Source: CAD feature listing. Evaluate the final solid. Frame: model axes, mm. A direction names the side the tool comes from. Give positions to 0.01 mm unless a question says otherwise; leave off trailing zeros. Loops run counter-clockwise (first coordinate to the right, second up) from the corner with the lowest first, then second, coordinate; pieces in that order, holes last. Notation, with made-up numbers: M 72.5,31.25 L 95.5,31.25 A21 cw 95.5,67.25 Z; hole C 13,-16 d3. An arc over 180 degrees is marked long. Answer in a Markdown table with one row per item.
```python
from build123d import *

# Parameters (mm, degrees)
SKETCH_5_W                = 42.3
SKETCH_5_H                = 50.3
SKETCH_5_R                = 11.15
SKETCH_5_R_2              = 2.15
EXTRUDE_2_DEPTH           = 4
EXTRUDE_3_DEPTH           = 4
SKETCH_7_R                = 1.7
CUT_EXTRUDE_3_DEPTH       = 4
CHAMFER_1_SIZE            = 4
EXTRUDE_4_DEPTH           = 2
EXTRUDE_5_REACH           = 79.8
EXTRUDE_6_REACH           = 80.956
SKETCH_12_W               = 46.3
SKETCH_12_H               = 3
EXTRUDE_7_DEPTH           = 53
EXTRUDE_9_DEPTH           = 4
CUT_EXTRUDE_4_DEPTH       = 5
SKETCH_17_R               = 5.175
EXTRUDE_10_DEPTH          = 15
SKETCH_18_R               = 1.6
CUT_EXTRUDE_6_DEPTH       = 15
F_2_0MM_1_D               = 3.1
F_2_0MM_1_DEPTH           = 4.45
F_2_0MM_1_TIP             = 1.55
F_2_0MM_1_ON_FACE_2_D     = 3.1
F_2_0MM_1_ON_FACE_2_DEPTH = 4.45
F_2_0MM_1_ON_FACE_2_TIP   = 1.55
F_2_0MM_1_ON_FACE_3_D     = 3.1
F_2_0MM_1_ON_FACE_3_DEPTH = 4.45
F_2_0MM_1_ON_FACE_3_TIP   = 1.55
SKETCH_21_W               = 46.3
SKETCH_21_H               = 53
CUT_EXTRUDE_7_DEPTH       = 1.5
CUT_EXTRUDE_START         = -0.5
CUT_EXTRUDE_8_DEPTH       = 0.5
EXTRUDE_START             = 2.5
EXTRUDE_11_DEPTH          = 2.5


with BuildPart() as part:
    # Sketch 5 → Extrude 2 (new body)
    with BuildSketch(Plane.XY):
        with Locations((0, 25.15)):
            Rectangle(SKETCH_5_W, SKETCH_5_H)
        with Locations((0, 29.15)):
            Circle(SKETCH_5_R, mode=Mode.SUBTRACT)
        with Locations((15.5, 44.65)):
            Circle(SKETCH_5_R_2, mode=Mode.SUBTRACT)
        with Locations(Location((15.5, 13.65, 0), (0, 0, 180))):
            Circle(SKETCH_5_R_2, mode=Mode.SUBTRACT)
        with Locations((-15.5, 13.65)):
            Circle(SKETCH_5_R_2, mode=Mode.SUBTRACT)
        with Locations(Location((-15.5, 44.65, 0), (0, 0, 180))):
            Circle(SKETCH_5_R_2, mode=Mode.SUBTRACT)
    extrude(amount=-EXTRUDE_2_DEPTH)

    # Sketch 6 → Extrude 3 (add)
    with BuildSketch(Plane.XZ):
        with BuildLine():
            Line((-21.15, 0), (-19.967256346, 20.643972909))
            ThreePointArc((-19.967256346, 20.643972909), (0, 39.5), (19.967256346, 20.643972909))
            Line((19.967256346, 20.643972909), (21.15, 0))
            Line((21.15, 0), (-21.15, 0))
        make_face()
    extrude(amount=-EXTRUDE_3_DEPTH)

    # Sketch 7 → Cut-Extrude 3 (cut)
    with BuildSketch(Plane(origin=(0, 4, 0), x_dir=(1, 0, 0), z_dir=(0, 1, 0))):
        with Locations(Location((0, -5.5, 0), (0, 0, 270))):
            Circle(SKETCH_7_R)
        with Locations(Location((12.124355653, -12.5, 0), (0, 0, 270))):
            Circle(SKETCH_7_R)
        with Locations(Location((12.124355653, -26.5, 0), (0, 0, 270))):
            Circle(SKETCH_7_R)
        with Locations(Location((0, -33.5, 0), (0, 0, 270))):
            Circle(SKETCH_7_R)
        with Locations(Location((-12.124355653, -26.5, 0), (0, 0, 270))):
            Circle(SKETCH_7_R)
        with Locations(Location((-12.124355653, -12.5, 0), (0, 0, 270))):
            Circle(SKETCH_7_R)
    extrude(amount=-CUT_EXTRUDE_3_DEPTH, mode=Mode.SUBTRACT)

    # Chamfer 1
    chamfer_1_edges = [part.edges().sort_by_distance(p)[0] for p in [
        (-21.15, 50.3, -2),
        (21.15, 50.3, -2),
    ]]
    chamfer(chamfer_1_edges, length=CHAMFER_1_SIZE)

    # Sketch 9 → Extrude 4 (add)
    with BuildSketch(Plane.ZY.offset(21.15)):
        Polygon((-4, 0), (8, 0), (2, 15.3), (-4, 15.3), align=None)
    extrude_4 = extrude(amount=EXTRUDE_4_DEPTH)

    # Extrude 5: up to this face of the body (flat: up to its plane)
    extrude_5_end = Plane(part.part.faces().sort_by_distance((-20.558628173, 2, 10.321986454))[0])
    # Sketch 10 → Extrude 5 (add, up to the picked face)
    with BuildSketch(Plane.ZY.offset(23.15), mode=Mode.PRIVATE) as extrude_5_sk1:
        Polygon((-4, 0), (8, 0), (6.431372549, 4), (-4, 4), align=None)
    extrude_5_tool1 = split(extrude(extrude_5_sk1.sketch, amount=-EXTRUDE_5_REACH, mode=Mode.PRIVATE), bisect_by=extrude_5_end, keep=Keep.BOTH, mode=Mode.PRIVATE)
    add(extrude_5_tool1.solids().sort_by(Axis((-23.15, 1.95338, 1.616984), (1, 0, 0)))[0])

    # Mirror 2: Extrude 4 across plane
    add(extrude_4.mirror(Plane(origin=(0, 0, 0), x_dir=(0, 0, 1), z_dir=(1, 0, 0))))

    # Extrude 6: up to this face of the body (flat: up to its plane)
    extrude_6_end = Plane(part.part.faces().sort_by_distance((20.558628173, 2, 10.321986454))[0])
    # Sketch 11 → Extrude 6 (add, up to the picked face)
    with BuildSketch(Plane(origin=(23.15, 0, 0), x_dir=(0, 0, -1), z_dir=(1, 0, 0)), mode=Mode.PRIVATE) as extrude_6_sk1:
        Polygon((-6.431372549, 4), (4, 4), (4, 0), (-8, 0), align=None)
    extrude_6_tool1 = split(extrude(extrude_6_sk1.sketch, amount=-EXTRUDE_6_REACH, mode=Mode.PRIVATE), bisect_by=extrude_6_end, keep=Keep.BOTH, mode=Mode.PRIVATE)
    add(extrude_6_tool1.solids().sort_by(Axis((23.15, 1.95338, 1.616984), (-1, 0, 0)))[0])

    # Sketch 12 → Extrude 7 (add)
    with BuildSketch(Plane(origin=(0, 0, -4), x_dir=(-1, 0, 0), z_dir=(0, 0, -1))):
        with Locations((0, 6.5)):
            Rectangle(SKETCH_12_W, SKETCH_12_H)
    extrude(amount=EXTRUDE_7_DEPTH)

    # Sketch 14 → Extrude 9 (add)
    with BuildSketch(Plane(origin=(0, 4, 0), x_dir=(1, 0, 0), z_dir=(0, 1, 0))):
        with BuildLine():
            Line((21.15, 0), (-21.15, 0))
            Line((-21.15, 0), (-21.15, -6.431372549))
            Line((-21.15, -6.431372549), (-20.781530951, -6.431372549))
            Line((-20.781530951, -6.431372549), (-19.967256346, -20.643972909))
            ThreePointArc((-19.967256346, -20.643972909), (0, -39.5), (19.967256346, -20.643972909))
            Line((19.967256346, -20.643972909), (20.781530951, -6.431372549))
            Line((20.781530951, -6.431372549), (21.15, -6.431372549))
            Line((21.15, -6.431372549), (21.15, 0))
        make_face()
    extrude(amount=EXTRUDE_9_DEPTH)

    # Sketch 15 → Cut-Extrude 4 (cut)
    with BuildSketch(Plane.XZ):
        with BuildLine():
            Line((-23.15, -4), (23.15, -4))
            Line((23.15, -4), (23.15, 8))
            Line((23.15, 8), (20.691660451, 8))
            Line((20.691660451, 8), (19.967256346, 20.643972909))
            ThreePointArc((19.967256346, 20.643972909), (0, 39.5), (-19.967256346, 20.643972909))
            Line((-19.967256346, 20.643972909), (-20.691660451, 8))
            Line((-20.691660451, 8), (-23.15, 8))
            Line((-23.15, 8), (-23.15, -4))
        make_face()
    extrude(amount=-CUT_EXTRUDE_4_DEPTH, mode=Mode.SUBTRACT)

    # Sketch 17 → Extrude 10 (add)
    with BuildSketch(Plane(origin=(0, 8, 0), x_dir=(1, 0, 0), z_dir=(0, 1, 0))):
        with Locations(Location((0, 16.5, 0), (0, 0, 270))):
            Circle(SKETCH_17_R)
    extrude(amount=-EXTRUDE_10_DEPTH)

    # Sketch 18 → Cut-Extrude 6 (cut)
    with BuildSketch(Plane.XZ.offset(7)):
        with Locations(Location((0, -16.5, 0), (0, 0, 270))):
            Circle(SKETCH_18_R)
    extrude(amount=-CUT_EXTRUDE_6_DEPTH, mode=Mode.SUBTRACT)

    # 2.0mm _1
    with Locations(Plane(origin=(-2.383959963, -1.470142013, -11.906813753), x_dir=(0.887572221549, 0, 0.46066859187), z_dir=(-0.46066859187, 0, 0.887572221549))):
        with Locations((0, 0)):
            Hole(F_2_0MM_1_D / 2, depth=F_2_0MM_1_DEPTH)
            with Locations((0, 0, -(F_2_0MM_1_DEPTH + F_2_0MM_1_TIP / 2))):  # 90° drill point
                Cone(0, F_2_0MM_1_D / 2, F_2_0MM_1_TIP, mode=Mode.SUBTRACT)

    # 2.0mm _1 on face 2
    with Locations(Plane(origin=(-4.001379199, -1.359919587, -19.781705274), x_dir=(0.634146160856, 0, -0.773213196131), z_dir=(-0.773213196131, 0, -0.634146160856))):
        with Locations((-1e-09, 0)):
            Hole(F_2_0MM_1_ON_FACE_2_D / 2, depth=F_2_0MM_1_ON_FACE_2_DEPTH)
            with Locations((0, 0, -(F_2_0MM_1_ON_FACE_2_DEPTH + F_2_0MM_1_ON_FACE_2_TIP / 2))):  # 90° drill point
                Cone(0, F_2_0MM_1_ON_FACE_2_D / 2, F_2_0MM_1_ON_FACE_2_TIP, mode=Mode.SUBTRACT)

    # 2.0mm _1 on face 3
    with Locations(Plane(origin=(4.74207792, -1.268589172, -18.572033301), x_dir=(0.40039282367, 0, 0.916343596449), z_dir=(0.916343596449, 0, -0.40039282367))):
        with Locations((0, 0)):
            Hole(F_2_0MM_1_ON_FACE_3_D / 2, depth=F_2_0MM_1_ON_FACE_3_DEPTH)
            with Locations((0, 0, -(F_2_0MM_1_ON_FACE_3_DEPTH + F_2_0MM_1_ON_FACE_3_TIP / 2))):  # 90° drill point
                Cone(0, F_2_0MM_1_ON_FACE_3_D / 2, F_2_0MM_1_ON_FACE_3_TIP, mode=Mode.SUBTRACT)

    # Sketch 21 → Cut-Extrude 7 (cut)
    with BuildSketch(Plane(origin=(0, 8, 0), x_dir=(1, 0, 0), z_dir=(0, 1, 0))):
        with Locations((0, 30.5)):
            Rectangle(SKETCH_21_W, SKETCH_21_H)
    extrude(amount=-CUT_EXTRUDE_7_DEPTH, mode=Mode.SUBTRACT)

    # Sketch 22 → Cut-Extrude 8 (cut)
    with BuildSketch(Plane(origin=(0, 8, 0), x_dir=(1, 0, 0), z_dir=(0, 1, 0)).offset(CUT_EXTRUDE_START)):
        with BuildLine():
            Line((21.15, -6.431372549), (21.15, -4.862745098))
            Line((21.15, -4.862745098), (21.15, 0))
            Line((21.15, 0), (-21.15, 0))
            Line((-21.15, 0), (-21.15, -4.862745098))
            Line((-21.15, -4.862745098), (-21.15, -6.431372549))
            Line((-21.15, -6.431372549), (-20.781530951, -6.431372549))
            Line((-20.781530951, -6.431372549), (-19.967256346, -20.643972909))
            ThreePointArc((-19.967256346, -20.643972909), (0, -39.5), (19.967256346, -20.643972909))
            Line((19.967256346, -20.643972909), (20.781530951, -6.431372549))
            Line((20.781530951, -6.431372549), (21.15, -6.431372549))
        make_face()
    extrude(amount=CUT_EXTRUDE_8_DEPTH, mode=Mode.SUBTRACT)

    # Sketch 23 → Extrude 11 (add)
    with BuildSketch(Plane.XZ.offset(-5).offset(EXTRUDE_START)):
        with BuildLine():
            Line((23.15, -57), (23.15, 6.039215686))
            Line((23.15, 6.039215686), (21.15, 6.039215686))
            Line((21.15, 6.039215686), (21.15, 6.431372549))
            Line((21.15, 6.431372549), (20.781530951, 6.431372549))
            Line((20.781530951, 6.431372549), (19.967256346, 20.643972909))
            ThreePointArc((19.967256346, 20.643972909), (0, 39.5), (-19.967256346, 20.643972909))
            Line((-19.967256346, 20.643972909), (-20.781530951, 6.431372549))
            Line((-20.781530951, 6.431372549), (-21.15, 6.431372549))
            Line((-21.15, 6.431372549), (-21.15, 6.039215686))
            Line((-21.15, 6.039215686), (-23.15, 6.039215686))
            Line((-23.15, 6.039215686), (-23.15, -57))
            Line((-23.15, -57), (23.15, -57))
        make_face()
    extrude(amount=-EXTRUDE_11_DEPTH)


solid = part.part
```
1) Pin query (flat end, axial travel): pin 1 Ø23 at (x, z) = (2, -42.5) entering from +Y; pin 2 Ø2 at (x, y) = (-22, 4) entering from +Z; pin 3 Ø2.5 at (x, z) = (0, -16.5) entering from +Y; pin 4 Ø3.5 at (x, y) = (15.5, 13.65) entering from -Z. Return the tip coordinate at first contact, or that it passes through.
Reply:
| item | result |
|---|---|
| pin 1 | stops at y = 6.5 |
| pin 2 | stops at z = 6.43 |
| pin 3 | stops at y = 5 |
| pin 4 | passes through |
2) Section D-D, the plane y = 44.65. Return loops of the section in (x, z).
Reply:
| item | result |
|---|---|
| outline | M -21.15,-4 L -17.65,-4 L -17.65,0 L -21.15,0 Z; M -13.35,-4 L 13.35,-4 L 13.35,0 L -13.35,0 Z; M 17.65,-4 L 21.15,-4 L 21.15,0 L 17.65,0 Z |
3) Pull-direction query (Y, two-part tool) for faces 6 (the flat face through (22, 4, 6.039)), 7 (the flat face through (0, 50.3, -2)), 8 (the cylindrical face through (-2.417, 18.265, -1.972)); classes: released by +Y, released by -Y, zero draft, split by the parting line, or undercut.
Reply:
| item | result |
|---|---|
| face 6 | zero draft |
| face 7 | released by +Y |
| face 8 | undercut |
4) Material intervals for L1, parallel to Y at x = 15.5, z = -1.4; L2, parallel to Y at x = 3, z = 25; L3, parallel to X at y = 13, z = -3, sorted ascending.
Reply:
| item | result |
|---|---|
| L1 | y = 2.5 to 11.5, 15.8 to 42.5, 46.8 to 50.3 |
| L2 | y = 2.5 to 7.5 |
| L3 | x = -23.15 to -17.55, -13.45 to 13.45, 17.55 to 23.15 |
5) Section C-C, the plane x = -10. Return loops of the section in (y, z), then the cut area to 3 significant figures.
Reply:
| item | result |
|---|---|
| outline | M 2.5,-57 L 6.5,-57 L 6.5,-4 L 24.22,-4 L 24.22,0 L 7.5,0 L 7.5,36.82 L 2.5,36.82 Z; M 34.08,-4 L 50.3,-4 L 50.3,0 L 34.08,0 Z |
| area | 548 mm² |
6) Section A-A, the plane y = 29.15. Return loops of the section in (x, z), then the cut area to 3 significant figures.
Reply:
| item | result |
|---|---|
| outline | M -21.15,-4 L -11.15,-4 L -11.15,0 L -21.15,0 Z; M 11.15,-4 L 21.15,-4 L 21.15,0 L 11.15,0 Z |
| area | 80.0 mm² |
7) Set-up query: faces 1 (the flat face through (-22, 4, 6.039)), 2 (the flat face through (-5, 19, -4)), 3 (the flat face through (0, 7.5, 19)), 4 (the cylindrical face through (1.08, -2.32, -15.32)), 5 (the flat face through (-22.136, 10.078, 4.048)). Return all of +Z, -Z, +X, -X, +Y, -Y with unobstructed straight access to the full face (end or side cutting, diameter ignored); none if empty.
Reply:
| item | result |
|---|---|
| face 1 | +Z, -X, +Y, -Y |
| face 2 | -Z, +X, -X, +Y |
| face 3 | +Z, +Y |
| face 4 | -Y |
| face 5 | +Z, -X, +Y |
8) Section B-B, the plane z = -2.5. Return loops of the section in (x, y).
Reply:
| item | result |
|---|---|
| outline | M -23.15,2.5 L 23.15,2.5 L 23.15,15.3 L 21.15,15.3 L 21.15,46.3 L 17.15,50.3 L -17.15,50.3 L -21.15,46.3 L -21.15,15.3 L -23.15,15.3 Z; hole C -15.5,13.65 d4.3; hole C -15.5,44.65 d4.3; hole C 0,29.15 d22.3; hole C 15.5,13.65 d4.3; hole C 15.5,44.65 d4.3 |
